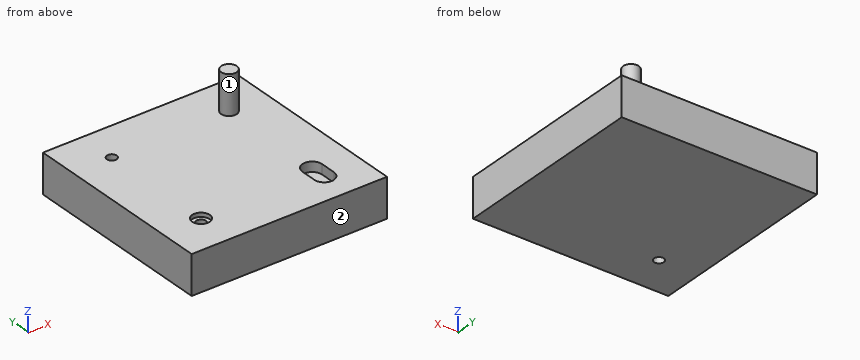
```python
from build123d import *

# Parameters (mm, degrees)
SKIZZE1_W                       = 100
SKIZZE1_H                       = 100
AUFSATZ_LINEAR_AUSTRAGEN1_DEPTH = 20
F_5_0MM_STIFTLOCH1_D            = 5
F_5_0MM_STIFTLOCH1_DEPTH        = 8.5
F_5_0MM_STIFTLOCH1_TIP          = 1.502151548
SKIZZE5_R                       = 4
AUFSATZ_LINEAR_AUSTRAGEN2_DEPTH = 20
BOHRUNG1_D                      = 5
BOHRUNG1_DEPTH                  = 20
BOHRUNG1_CBORE_D                = 9
BOHRUNG1_CBORE_DEPTH            = 2.1
BOHRUNG1_TIP                    = 1.502151548
SCHNITT_LINEAR_AUSTRAGEN1_DEPTH = 5


with BuildPart() as part:
    # Skizze1 → Aufsatz-Linear austragen1 (new body)
    with BuildSketch(Plane.XY):
        Rectangle(SKIZZE1_W, SKIZZE1_H)
    extrude(amount=AUFSATZ_LINEAR_AUSTRAGEN1_DEPTH)

    # Ø5.0mm Stiftloch1
    with Locations(Plane.XY.offset(20)):
        with Locations((-30, 30)):
            Hole(F_5_0MM_STIFTLOCH1_D / 2, depth=F_5_0MM_STIFTLOCH1_DEPTH)
            with Locations((0, 0, -(F_5_0MM_STIFTLOCH1_DEPTH + F_5_0MM_STIFTLOCH1_TIP / 2))):  # 118° drill point
                Cone(0, F_5_0MM_STIFTLOCH1_D / 2, F_5_0MM_STIFTLOCH1_TIP, mode=Mode.SUBTRACT)

    # Skizze5 → Aufsatz-Linear austragen2 (add)
    with BuildSketch(Plane.XY.offset(20)):
        with Locations(Location((30, 30, 0), (0, 0, 180))):
            Circle(SKIZZE5_R)
    extrude(amount=AUFSATZ_LINEAR_AUSTRAGEN2_DEPTH)

    # Bohrung1
    with Locations(Plane.XY.offset(20)):
        with Locations((-30, -30)):
            CounterBoreHole(BOHRUNG1_D / 2, BOHRUNG1_CBORE_D / 2, BOHRUNG1_CBORE_DEPTH, depth=BOHRUNG1_DEPTH)
            with Locations((0, 0, -(BOHRUNG1_DEPTH + BOHRUNG1_TIP / 2))):  # 118° drill point
                Cone(0, BOHRUNG1_D / 2, BOHRUNG1_TIP, mode=Mode.SUBTRACT)

    # Skizze9 → Schnitt-Linear austragen1 (cut)
    with BuildSketch(Plane.XY.offset(20)):
        with BuildLine():
            Line((25, -34), (25, -26))
            ThreePointArc((25, -26), (30, -21), (35, -26))
            Line((35, -26), (35, -34))
            ThreePointArc((35, -34), (30, -39), (25, -34))
        make_face()
    extrude(amount=-SCHNITT_LINEAR_AUSTRAGEN1_DEPTH, mode=Mode.SUBTRACT)


solid = part.part
```
The listing builds one solid part. Answer for the finished solid, in the listing's coordinates (mm). Face numbers are marked on the shaded views. A direction names the side the tool comes from. Give positions to 0.01 mm unless a question says otherwise; leave off trailing zeros. Loops run counter-clockwise (first coordinate to the right, second up) from the corner with the lowest first, then second, coordinate; pieces in that order, holes last. Notation, with made-up numbers: (50, -1) - (71, -1) arc R25 ccw to (71, 34) - close; hole circle Ø11 at (83.25, 1.25). An arc over 180 degrees is marked (long way). Answer as CSV lines item,"result". Start each with the question number.
Item 1: A cutting plane is placed at A-A on x = 30. Determine the outline of the cut face in (y, z), then the cut area to 3 significant figures.
Item 2: A cutting plane is placed at C-C on y = 24. Determine the outline of the cut face in (x, z), then the cut area to 3 significant figures.
Item 3: For the marked faces 1 and 2, determine the directions among +Z, -Z, +X, -X, +Y, -Y from which every point of the face is accessible in a straight line to the end or side of a thin tool.
Item 4: Each of these flat-tipped pins is pushed along its axis until it touches: pin 1 (3 mm diameter, centred on x = 31.5, y = -34, fed in from +Z); pin 2 (4 mm diameter, centred on x = -30, y = -30, fed in from +Z); pin 3 (3 mm diameter, centred on x = -37, y = 14.5, fed in from +Z); pin 4 (4.5 mm diameter, centred on x = -31, y = -30.5, fed in from +Z). Where does it stop, or does it pass through?
Item 5: A cutting plane is placed at B-B on z = 22. Determine the outline of the cut face in (x, y).
Item 6: Find the intervals of material crossed by line 1 (X direction, y = -30, z = 13); line 2 (Y direction, x = -30, z = 17.5), in increasing order. Write a range as from..to.
Found:
1,outline,"(-50, 0) - (50, 0) - (50, 20) - (34, 20) - (34, 40) - (26, 40) - (26, 20) - (-21, 20) - (-21, 15) - (-39, 15) - (-39, 20) - (-50, 20) - close"
1,area,"2,070 mm^2"
2,outline,"(-50, 0) - (50, 0) - (50, 20) - (-50, 20) - close"
2,area,"2,000 mm^2"
3,face 1,"+Z"
3,face 2,"+Z, -Z, +X, -X, -Y"
4,pin 1,"stops at z = 15"
4,pin 2,"passes through"
4,pin 3,"stops at z = 20"
4,pin 4,"stops at z = 17.9"
5,outline,"circle Ø8 at (30, 30)"
6,line 1,"x = -50..-32.5, -27.5..50"
6,line 2,"y = -50..-32.5, -27.5..27.5, 32.5..50"
